from build123d import *

# Parameters (mm, degrees)
F0_W     = 280.5716638824
F0_H     = 260.4053167929
F1_DEPTH = 6.35
F2_D     = 7.9756


with BuildPart() as f1:
    # F0 (on Front) → F1 (new body)
    with BuildSketch(Plane.XZ):
        with Locations((0, 21.7262194655)):
            Rectangle(F0_W, F0_H)
        with BuildLine():
            ThreePointArc((-75.2618319412, -51.326438931), (-82.0809159706, -47.389438931), (-82.0809159706, -39.515438931))
            Line((-82.0809159706, -39.515438931), (-6.8190840294, 90.8418778619))
            ThreePointArc((-6.8190840294, 90.8418778619), (0, 94.7788778619), (6.8190840294, 90.8418778619))
            Line((6.8190840294, 90.8418778619), (82.0809159706, -39.515438931))
            ThreePointArc((82.0809159706, -39.515438931), (82.0809159706, -47.389438931), (75.2618319412, -51.326438931))
            Line((75.2618319412, -51.326438931), (-75.2618319412, -51.326438931))
        make_face(mode=Mode.SUBTRACT)
        with BuildLine():
            Line((-6.8190840294, 90.8418778619), (-82.0809159706, -39.515438931))
            ThreePointArc((-82.0809159706, -39.515438931), (-82.0809159706, -47.389438931), (-75.2618319412, -51.326438931))
            Line((-75.2618319412, -51.326438931), (75.2618319412, -51.326438931))
            ThreePointArc((75.2618319412, -51.326438931), (82.0809159706, -47.389438931), (82.0809159706, -39.515438931))
            Line((82.0809159706, -39.515438931), (6.8190840294, 90.8418778619))
            ThreePointArc((6.8190840294, 90.8418778619), (0, 94.7788778619), (-6.8190840294, 90.8418778619))
        make_face()
    extrude(amount=F1_DEPTH)

    # F2 (through all)
    with Locations(Plane(origin=(0, 0, 0), x_dir=(1, 0, 0), z_dir=(0, 1, 0))):
        with Locations((0, -86.9048778619), (-75.2618319412, 43.452438931), (75.2618319412, 43.452438931)):
            Hole(F2_D / 2)


solid = f1.part
Can you work these out from the model? Positions are in its coordinate system, mm. Give positions to 0.01 mm unless a question says otherwise; leave off trailing zeros. Loops run counter-clockwise (first coordinate to the right, second up) from the corner with the lowest first, then second, coordinate; pieces in that order, holes last. Notation, with made-up numbers: (85, -4) -> (127, -4) arc R16 ccw to (127, 9) -> close; hole circle Ø2 at (9.25, 22). An arc over 180 degrees is marked (long way). Return JSON: item names as keys, results as strings.
Q1. I want a section at A-A, the plane x = 0. List the corners of the cut face in (y, z) for me, then the cut area to 3 significant figures.
Checks:
{"outline": "(-6.35, -108.48) -> (0, -108.48) -> (0, 82.92) -> (-6.35, 82.92) -> close; (-6.35, 90.89) -> (0, 90.89) -> (0, 151.93) -> (-6.35, 151.93) -> close", "area": "1,600 mm2"}
Q2. I need wall thicknesses on probe 1 along X at (y, z) = (-6, -41.5); probe 2 along Z at (x, y) = (0, -4.75); probe 3 along X at (y, z) = (-4.5, -44.5). Which ranges of each line are inside material? Lowest first, please.
Checks:
{"probe 1": "x = -140.29 to -78.74, -71.78 to 71.78, 78.74 to 140.29", "probe 2": "z = -108.48 to 82.92, 90.89 to 151.93", "probe 3": "x = -140.29 to -79.11, -71.41 to 71.41, 79.11 to 140.29"}
Q3. We'd pull the mould along Z, two halves only. Please class faces 1 (the face through (-140.286, -3, 20)), 2 (the face through (-72.097, -3.219, -41.026)), 3 (the face through (-2, -3, -108.476)): released by +Z, released by -Z, zero draft, split by the parting line, or undercut.
Checks:
{"face 1": "zero draft", "face 2": "undercut", "face 3": "released by -Z"}
